from build123d import *

# Parameters (mm, degrees)
F1_DEPTH = 25


with BuildPart() as f1:
    # F0 (on Top) → F1 (new body)
    with BuildSketch(Plane.XY):
        Polygon((-104.5, 104.1464466094), (-105, 104.6464466094), (-105, -104.6464466094), (-104.5, -104.1464466094), align=None)
        Polygon((-104.1464466094, -104.5), (-104.6464466094, -105), (104.6464466094, -105), (104.1464466094, -104.5), align=None)
        Polygon((-104.5, -104.5), (-105, -105), (-104.6464466094, -105), (-104.1464466094, -104.5), align=None)
        Polygon((-104.5, -104.1464466094), (-105, -104.6464466094), (-105, -105), (-104.5, -104.5), align=None)
        Polygon((-0.1767766953, -0.1767766953), (-104.5, -104.5), (-104.1464466094, -104.5), (0, -0.3535533906), align=None)
        Polygon((-0.3535533906, 0), (-104.5, -104.1464466094), (-104.5, -104.5), (-0.1767766953, -0.1767766953), align=None)
        Polygon((105, -104.6464466094), (105, 104.6464466094), (104.5, 104.1464466094), (104.5, -104.1464466094), align=None)
        Polygon((105, -105), (105, -104.6464466094), (104.5, -104.1464466094), (104.5, -104.5), align=None)
        Polygon((104.1464466094, -104.5), (104.6464466094, -105), (105, -105), (104.5, -104.5), align=None)
        Polygon((104.5, -104.5), (0.1767766953, -0.1767766953), (0, -0.3535533906), (104.1464466094, -104.5), align=None)
        Polygon((0.3535533906, 0), (0.1767766953, -0.1767766953), (104.5, -104.5), (104.5, -104.1464466094), align=None)
        Polygon((0, 0), (-0.1767766953, 0.1767766953), (-0.3535533906, 0), (-0.1767766953, -0.1767766953), align=None)
        Polygon((0.1767766953, -0.1767766953), (0, 0), (-0.1767766953, -0.1767766953), (0, -0.3535533906), align=None)
        Polygon((0.1767766953, 0.1767766953), (0, 0), (0.1767766953, -0.1767766953), (0.3535533906, 0), align=None)
        Polygon((0, 0.3535533906), (-0.1767766953, 0.1767766953), (0, 0), (0.1767766953, 0.1767766953), align=None)
        Polygon((104.5, 104.1464466094), (104.5, 104.5), (0.1767766953, 0.1767766953), (0.3535533906, 0), align=None)
        Polygon((104.5, 104.5), (104.1464466094, 104.5), (0, 0.3535533906), (0.1767766953, 0.1767766953), align=None)
        Polygon((-104.1464466094, 104.5), (-104.5, 104.5), (-0.1767766953, 0.1767766953), (0, 0.3535533906), align=None)
        Polygon((-0.1767766953, 0.1767766953), (-104.5, 104.5), (-104.5, 104.1464466094), (-0.3535533906, 0), align=None)
        Polygon((-104.5, 104.5), (-105, 105), (-105, 104.6464466094), (-104.5, 104.1464466094), align=None)
        Polygon((-104.6464466094, 105), (-105, 105), (-104.5, 104.5), (-104.1464466094, 104.5), align=None)
        Polygon((104.6464466094, 105), (-104.6464466094, 105), (-104.1464466094, 104.5), (104.1464466094, 104.5), align=None)
        Polygon((105, 105), (104.6464466094, 105), (104.1464466094, 104.5), (104.5, 104.5), align=None)
        Polygon((105, 104.6464466094), (105, 105), (104.5, 104.5), (104.5, 104.1464466094), align=None)
    extrude(amount=F1_DEPTH)


solid = f1.part
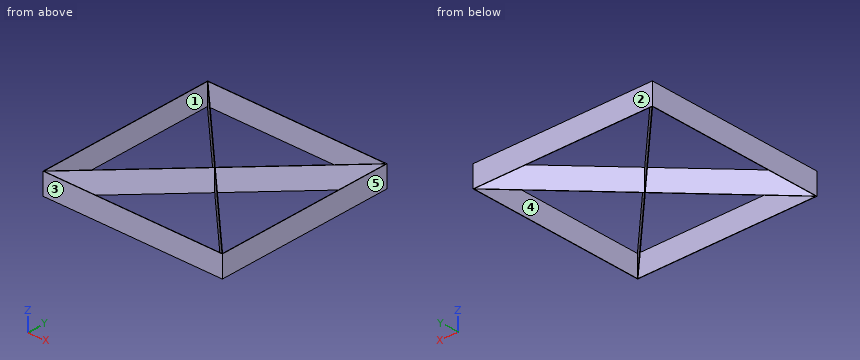
The listing builds one solid part. Answer for the finished solid, in the listing's coordinates (mm). Face numbers are marked on the shaded views. A direction names the side the tool comes from. Give positions to 0.01 mm unless a question says otherwise; leave off trailing zeros. Write each loop counter-clockwise with the first axis right and the second up, starting at its lowest first coordinate (ties: lowest second). Pieces come first, ordered by that corner, then holes.
Item 1: Determine the mould class of the marked faces 3, 4 and 5 for opening direction Y: released by +Y, released by -Y, zero draft, split by the parting line, or undercut.
Item 2: Section B-B, the plane y = -74.5 is taken. Write down the section's boundary in (x, z).
Item 3: Find the intervals of material crossed by line 1 along X through (y, z) = (13.5, 16); line 2 along Y through (x, z) = (71, 13.25); line 3 along X through (y, z) = (-69, 21.5), in increasing order.
Item 4: Section A-A, the plane z = 20.25 is taken. Write down the section's boundary in (x, y), plus the area to 3 significant figures.
Item 5: Section C-C, the plane x = 77.5 is taken. Write down the section's boundary in (y, z), plus the area to 3 significant figures.
Item 6: Which of the six approach directions +Z, -Z, +X, -X, +Y, -Y give full straight-line access (tool end or side, diameter ignored) to the marked faces 1 and 2?
Completed:
1. face 3: released by -Y
1. face 4: undercut
1. face 5: zero draft
2. outline: (-105, 0) - (-104.5, 0) - (-104.5, 25) - (-105, 25) - close; (-74.85, 0) - (-74.15, 0) - (-74.15, 25) - (-74.85, 25) - close; (74.15, 0) - (74.85, 0) - (74.85, 25) - (74.15, 25) - close; (104.5, 0) - (105, 0) - (105, 25) - (104.5, 25) - close
3. line 1: x = -105 to -104.5, -13.85 to -13.15, 13.15 to 13.85, 104.5 to 105
3. line 2: y = -105 to -104.5, -71.35 to -70.65, 70.65 to 71.35, 104.5 to 105
3. line 3: x = -105 to -104.5, -69.35 to -68.65, 68.65 to 69.35, 104.5 to 105
4. outline: (-105, -105) - (105, -105) - (105, 105) - (-105, 105) - close; hole (-104.5, -104.15) - (-0.35, 0) - (-104.5, 104.15) - close; hole (-104.15, -104.5) - (104.15, -104.5) - (0, -0.35) - close; hole (-104.15, 104.5) - (0, 0.35) - (104.15, 104.5) - close; hole (0.35, 0) - (104.5, -104.15) - (104.5, 104.15) - close
4. area: 714 mm2
5. outline: (-105, 0) - (-104.5, 0) - (-104.5, 25) - (-105, 25) - close; (-77.85, 0) - (-77.15, 0) - (-77.15, 25) - (-77.85, 25) - close; (77.15, 0) - (77.85, 0) - (77.85, 25) - (77.15, 25) - close; (104.5, 0) - (105, 0) - (105, 25) - (104.5, 25) - close
5. area: 60.4 mm2
6. face 1: +Z, -Z
6. face 2: +Z, -Z, +X, -X, +Y
